The model under review builds one solid part; all positions refer to its coordinate system, in mm. Coordinates: 2 decimals unless noted, no trailing zeros. Order: outer loops, then holes, each group sorted by start corner. A loop starts at its lowest first (then second) coordinate and runs counter-clockwise, first axis right, second up. Notation, with made-up numbers: (45.5, 52.5) -> (62.5, 52.5) arc R18 ccw to (62.5, 65.5) -> close; hole circle Ø9 at (-23, 84.25). An arc over 180 degrees is marked (long way). Put each result on its own line as item: value.
from build123d import *

# Parameters (mm, degrees)
SKETCH1_R           = 5.75
BOSS_EXTRUDE1_DEPTH = 3
BOSS_EXTRUDE2_DEPTH = 0.15
CIRPATTERN1_COUNT   = 2
SKETCH4_R           = 2.5
CUT_EXTRUDE1_DEPTH  = 65.47946021
CHAMFER1_SIZE       = 1


with BuildPart() as part:
    # Sketch1 → Boss-Extrude1 (new, symmetric)
    with BuildSketch(Plane(origin=(0, 0, 0), x_dir=(1, 0, 0), z_dir=(0, 1, 0))):
        with Locations(Location((0, 0, 0), (0, 0, 270))):
            Circle(SKETCH1_R)
    extrude(amount=BOSS_EXTRUDE1_DEPTH, both=True)

    # Sketch3 → Boss-Extrude2 (add, symmetric)
    with BuildSketch(Plane(origin=(0, 0, 0), x_dir=(0.9433030867471315, -0.3319326536111411, 0), z_dir=(-0.3319326536111411, -0.9433030867471315, 0))):
        with BuildLine():
            Line((-3.485399679, 3.239580817), (-6.069792392, 6.68067591))
            Line((-6.069792392, 6.68067591), (-6.069792392, 60.5))
            ThreePointArc((-6.069792392, 60.5), (-5.191112735, 62.621320344), (-3.069792392, 63.5))
            Line((-3.069792392, 63.5), (-2.854583135, 63.5))
            ThreePointArc((-2.854583135, 63.5), (0.220398514, 62.442649853), (1.994847243, 59.717795145))
            add(Edge.make_bspline(
                [(1.994847243, 59.717795145), (15.859721153, 31.612778986), (4.812953003, 1.848788557)],
                knots=[0, 0, 0, 1, 1, 1], degree=2))
            add(Edge.make_bspline(
                [(-3.485399679, 3.239580817), (0.91627292, 7.753975077), (4.812953003, 1.848788557)],
                knots=[0, 0, 0, 1, 1, 1], degree=2))
        make_face()
    boss_extrude2 = extrude(amount=BOSS_EXTRUDE2_DEPTH, both=True)

    # CirPattern1: Boss-Extrude2 ×2 about axis
    cirpattern1_axis = Axis((0, 3, 0), (0, -1, 0))
    for i in range(1, CIRPATTERN1_COUNT):
        add(boss_extrude2.rotate(cirpattern1_axis, i * 360 / CIRPATTERN1_COUNT))

    # Sketch4 → Cut-Extrude1 (cut, through all)
    with BuildSketch(Plane(origin=(0, 3, 0), x_dir=(1, 0, 0), z_dir=(0, 1, 0))):
        with Locations(Location((0, 0, 0), (0, 0, 270))):
            Circle(SKETCH4_R)
    extrude(amount=-CUT_EXTRUDE1_DEPTH, mode=Mode.SUBTRACT)

    # Chamfer1
    chamfer1_edges = [part.edges().sort_by_distance(p)[0] for p in [
        (0, -3, -2.5),
        (0, 3, -2.5),
    ]]
    chamfer(chamfer1_edges, length=CHAMFER1_SIZE)


solid = part.part
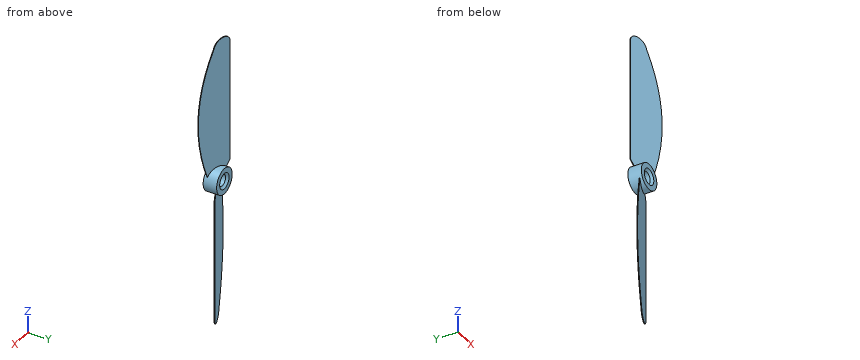
Item 1: Consider section A-A on z = 0. Write out the cut boundary in (x, y).
Answers below:
outline: (-5.75, -3) -> (-3.5, -3) -> (-2.5, -2) -> (-2.5, 2) -> (-3.5, 3) -> (-5.75, 3) -> close; (2.5, -2) -> (3.5, -3) -> (5.75, -3) -> (5.75, 3) -> (3.5, 3) -> (2.5, 2) -> close
Item 2: For line 1 (Z direction, x = 0, y = -2.5); line 2 (X direction, y = -0.1, z = 0); line 3 (Z direction, x = -2, y = -1.75), list the stretches that pass through material, from the lowest coordinate up. Write a range as from..to.
Answers below:
line 1: -5.75..-3, 3..5.75
line 2: -5.75..-2.5, 2.5..5.75
line 3: -5.39..-1.5, 1.5..5.39
Item 3: For pin 1 Ø4 at (x, z) = (5.5, -48.5) entering from +Y; pin 2 Ø3.5 at (x, z) = (-2.5, 1.5) entering from -Y; pin 3 Ø4 at (x, z) = (4, 7) entering from +Y, all flat-tipped, find the tip position at first contact; note any pin that passes through.
Answers below:
pin 1: y = 2.16
pin 2: y = -3
pin 3: y = -0.54
